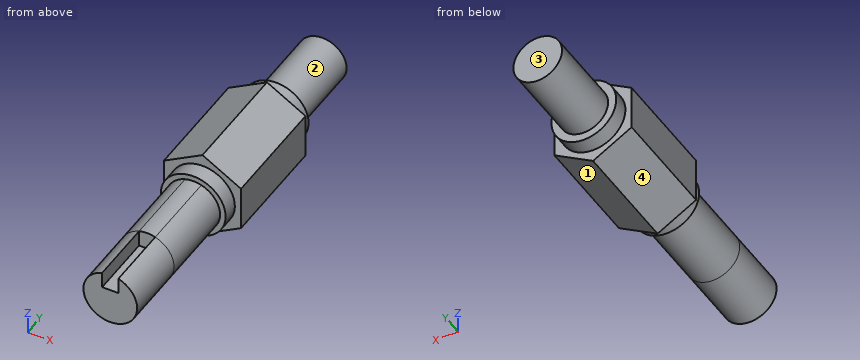
```python
from build123d import *

# Parameters (mm, degrees)
BOSS_EXTRUDE1_DEPTH = 14
SKETCH4_R           = 4
BOSS_EXTRUDE2_DEPTH = 2
SKETCH4_7_R         = 3.314528
BOSS_EXTRUDE3_DEPTH = 12
BOSS_EXTRUDE5_START = 2
SKETCH5_R           = 4
SKETCH5_R_2         = 3
BOSS_EXTRUDE5_DEPTH = 2
SKETCH5_4_R         = 3
BOSS_EXTRUDE6_DEPTH = 12
BOSS_EXTRUDE7_DEPTH = 20


with BuildPart() as part:
    # Sketch1 → Boss-Extrude1 (new body)
    with BuildSketch(Plane(origin=(0, 0, 0), x_dir=(1, 0, 0), z_dir=(0, 1, 0))):
        Polygon((4.7625, -2.749631), (4.7625, 2.749631), (0, 5.499261), (-4.7625, 2.749631), (-4.7625, -2.749631), (0, -5.499261), align=None)
    extrude(amount=BOSS_EXTRUDE1_DEPTH)

    # Sketch4 → Boss-Extrude2 (add)
    with BuildSketch(Plane.XZ):
        with Locations(Location((0, 0, 0), (0, 0, 270))):
            Circle(SKETCH4_R)
    extrude(amount=BOSS_EXTRUDE2_DEPTH)

    # Sketch4<7> → Boss-Extrude3 (add)
    with BuildSketch(Plane.XZ):
        with Locations(Location((0, 0, 0), (0, 0, 270))):
            Circle(SKETCH4_7_R)
        with BuildLine():
            Line((-1, 3.160079), (-1, 1.160079))
            Line((-1, 1.160079), (1, 1.160079))
            Line((1, 1.160079), (1, 3.160079))
            ThreePointArc((1, 3.160079), (0, -3.314528), (-1, 3.160079))
        make_face()
    extrude(amount=BOSS_EXTRUDE3_DEPTH)

    # Sketch5 → Boss-Extrude5 (add)
    # profile 1 of 2: a face of its own
    with BuildSketch(Plane(origin=(0, 14, 0), x_dir=(1, 0, 0), z_dir=(0, 1, 0)).offset(BOSS_EXTRUDE5_START)):
        with Locations(Location((0, 0, 0), (0, 0, 90))):
            Circle(SKETCH5_R)
        Circle(SKETCH5_R_2, mode=Mode.SUBTRACT)
    # profile 2 of 2: a face of its own
    with BuildSketch(Plane(origin=(0, 14, 0), x_dir=(1, 0, 0), z_dir=(0, 1, 0)).offset(BOSS_EXTRUDE5_START)):
        Circle(SKETCH5_R_2)
    extrude(amount=-BOSS_EXTRUDE5_DEPTH)

    # Sketch5<4> → Boss-Extrude6 (add)
    with BuildSketch(Plane(origin=(0, 14, 0), x_dir=(1, 0, 0), z_dir=(0, 1, 0))):
        with Locations(Location((0, 0, 0), (0, 0, 270))):
            Circle(SKETCH5_4_R)
    extrude(amount=BOSS_EXTRUDE6_DEPTH)

    # Sketch4<13> → Boss-Extrude7 (add)
    with BuildSketch(Plane.XZ):
        with BuildLine():
            Line((-1, 3.160079), (-1, 1.160079))
            Line((-1, 1.160079), (1, 1.160079))
            Line((1, 1.160079), (1, 3.160079))
            ThreePointArc((1, 3.160079), (0, -3.314528), (-1, 3.160079))
        make_face()
    extrude(amount=BOSS_EXTRUDE7_DEPTH)


solid = part.part
```
The listing builds one solid part. Answer for the finished solid, in the listing's coordinates (mm). Face numbers are marked on the shaded views. Coordinates: 2 decimals unless noted, no trailing zeros. Write each loop counter-clockwise with the first axis right and the second up, starting at its lowest first coordinate (ties: lowest second). Pieces come first, ordered by that corner, then holes. Notation, with made-up numbers: (71.25, 49) - (101.25, 49) arc R20 cw to (101.25, 71) - close; hole circle Ø11 at (-35.5, 29). An arc over 180 degrees is marked (long way). Return JSON: item names as keys, results as strings. Group by question number.
Q1. The part is cut by section B-B on x = -1.75. Write down the section's boundary in (y, z).
Q2. Find the intervals of material crossed by line 1 along Y through (x, z) = (-2.25, 3); line 2 along X through (y, z) = (24.5, 0); line 3 along Y through (x, z) = (-2.75, -3.75), in increasing order. Write a range as [from, to].
Q3. The part is cut by section D-D on z = 1.75. Write down the section's boundary in (x, y).
Q4. Flat-ended cylindrical pins translate along their axes: pin 1 Ø1.5 at (x, y) = (1, -5.5) entering from +Z; pin 2 Ø1.6 at (x, y) = (0, -15.5) entering from +Z; pin 3 Ø1 at (x, y) = (-2.5, 9) entering from +Z. Find the tip coordinate at first contact, or state that the pin passes through.
Q5. The part is cut by section A-A on z = 0. Write down the section's boundary in (x, y).
Q6. For a pull along X with two mould halves and no side action, classify the marked faces 1, 2, 3 and 4 as +X half, -X half, draft (parallel to the pull), parting line (faces both ways), or undercut.
Q7. The part is cut by section C-C on y = 3. Write down the section's boundary in (x, z).
Evaluation:
{
 "1": {"outline": "(-20, -2.81) - (-2, -2.81) - (-2, -3.6) - (0, -3.6) - (0, -4.49) - (14, -4.49) - (14, -3.6) - (16, -3.6) - (16, -2.44) - (26, -2.44) - (26, 2.44) - (16, 2.44) - (16, 3.6) - (14, 3.6) - (14, 4.49) - (0, 4.49) - (0, 3.6) - (-2, 3.6) - (-2, 2.81) - (-20, 2.81) - close"},
 "2": {"line 1": "y = [-2, 16]", "line 2": "x = [-3, 3]", "line 3": "y = [0, 14]"},
 "3": {"outline": "(-4.76, 0) - (-3.6, 0) - (-3.6, -2) - (-2.81, -2) - (-2.81, -20) - (-1, -20) - (-1, -12) - (1, -12) - (1, -20) - (2.81, -20) - (2.81, -2) - (3.6, -2) - (3.6, 0) - (4.76, 0) - (4.76, 14) - (3.6, 14) - (3.6, 16) - (2.44, 16) - (2.44, 26) - (-2.44, 26) - (-2.44, 16) - (-3.6, 16) - (-3.6, 14) - (-4.76, 14) - close"},
 "4": {"pin 1": "stops at z = 3.31", "pin 2": "stops at z = 1.16", "pin 3": "stops at z = 4.34"},
 "5": {"outline": "(-4.76, 0) - (-4, 0) - (-4, -2) - (-3.31, -2) - (-3.31, -20) - (3.31, -20) - (3.31, -2) - (4, -2) - (4, 0) - (4.76, 0) - (4.76, 14) - (4, 14) - (4, 16) - (3, 16) - (3, 26) - (-3, 26) - (-3, 16) - (-4, 16) - (-4, 14) - (-4.76, 14) - close"},
 "6": {"face 1": "+X half", "face 2": "parting line", "face 3": "draft", "face 4": "-X half"},
 "7": {"outline": "(-4.76, -2.75) - (0, -5.5) - (4.76, -2.75) - (4.76, 2.75) - (0, 5.5) - (-4.76, 2.75) - close"}
}
